Read the model definition and answer for the solid it produces. Units are mm, in the model's axes. A direction names the side the tool comes from. Coordinates: 2 decimals unless noted, no trailing zeros. Order: outer loops, then holes, each group sorted by start corner. A loop starts at its lowest first (then second) coordinate and runs counter-clockwise, first axis right, second up. Notation, with made-up numbers: M -10,24.5 L 20,24.5 A24 cw 20,38.5 Z; hole C -30,31.5 d8. An arc over 180 degrees is marked long. Put each result on its own line as item: value.
from build123d import *

# Parameters (mm, degrees)
F0_R         = 5.25
F1_DEPTH     = 30
F2_DEPTH     = 15
F3_DEPTH     = 30
F4_R         = 2
F6_DEPTH     = 22
F4_R_2       = 3.5
F7_DEPTH     = 4
F5_R         = 2
F8_DEPTH     = 4
F9_W         = 1
F9_H         = 30
F10_DEPTH    = 15
F11_T1_DEPTH = 80
F12_T1_DEPTH = 35.7073493424


# Not quite as in the source:
# - a fillet or chamfer that OpenCascade refuses, or shapes differently, is made with other operations: its cross-section is extruded or revolved along the edge and cut away or added


with BuildPart() as f1:
    # F0 (on Top) → F1 (new body)
    with BuildSketch(Plane.XY):
        with BuildLine():
            ThreePointArc((-11, 0), (0, -11), (11, 0))
            ThreePointArc((11, 0), (7.7781745931, 7.7781745931), (0, 11))
            ThreePointArc((0, 11), (-7.7781745931, 7.7781745931), (-11, 0))
        make_face()
        Circle(F0_R, mode=Mode.SUBTRACT)
        Circle(F0_R)
        with BuildLine():
            ThreePointArc((-1.5811388301, -2.25), (-1.2677476518, 2.4403515918), (2.75, 0))
            ThreePointArc((2.75, 0), (2.4403515918, -1.2677476518), (1.5811388301, -2.25))
            ThreePointArc((1.5811388301, -2.25), (0, -2.75), (-1.5811388301, -2.25))
        make_face(mode=Mode.SUBTRACT)
        with BuildLine():
            ThreePointArc((-11, 0), (-7.7781745931, 7.7781745931), (0, 11))
            Line((0, 11), (-11, 11))
            Line((-11, 11), (-11, 0))
        make_face()
        with BuildLine():
            ThreePointArc((0, 11), (7.7781745931, 7.7781745931), (11, 0))
            Line((11, 0), (11, 11))
            Line((11, 11), (0, 11))
        make_face()
        Polygon((-11, 11), (0, 11), (11, 11), (11, 13), (-11, 13), align=None)
        with BuildLine():
            Line((0, -2.25), (-1.5811388301, -2.25))
            ThreePointArc((-1.5811388301, -2.25), (0, -2.75), (1.5811388301, -2.25))
            Line((1.5811388301, -2.25), (0, -2.25))
        make_face()
        with BuildLine():
            ThreePointArc((1.5811388301, -2.25), (2.4403515918, -1.2677476518), (2.75, 0))
            ThreePointArc((2.75, 0), (-1.2677476518, 2.4403515918), (-1.5811388301, -2.25))
            Line((-1.5811388301, -2.25), (0, -2.25))
            Line((0, -2.25), (1.5811388301, -2.25))
        make_face()
    extrude(amount=F1_DEPTH)

    # F0 (on Top) → F2 (cut)
    with BuildSketch(Plane.XY):
        Circle(F0_R)
        with BuildLine():
            ThreePointArc((-1.5811388301, -2.25), (-1.2677476518, 2.4403515918), (2.75, 0))
            ThreePointArc((2.75, 0), (2.4403515918, -1.2677476518), (1.5811388301, -2.25))
            ThreePointArc((1.5811388301, -2.25), (0, -2.75), (-1.5811388301, -2.25))
        make_face(mode=Mode.SUBTRACT)
        with BuildLine():
            Line((0, -2.25), (-1.5811388301, -2.25))
            ThreePointArc((-1.5811388301, -2.25), (0, -2.75), (1.5811388301, -2.25))
            Line((1.5811388301, -2.25), (0, -2.25))
        make_face()
    extrude(amount=F2_DEPTH, mode=Mode.SUBTRACT)

    # F0 (on Top) → F3 (cut)
    with BuildSketch(Plane.XY):
        with BuildLine():
            ThreePointArc((1.5811388301, -2.25), (2.4403515918, -1.2677476518), (2.75, 0))
            ThreePointArc((2.75, 0), (-1.2677476518, 2.4403515918), (-1.5811388301, -2.25))
            Line((-1.5811388301, -2.25), (0, -2.25))
            Line((0, -2.25), (1.5811388301, -2.25))
        make_face()
    extrude(amount=F3_DEPTH, mode=Mode.SUBTRACT)

    # F4 (on face) → F6 (cut)
    with BuildSketch(Plane(origin=(-11, 0, 0), x_dir=(0, -1, 0), z_dir=(-1, 0, 0))):
        with Locations((-8, 7)):
            Circle(F4_R)
        with Locations((-8, 23)):
            Circle(F4_R)
    extrude(amount=-F6_DEPTH, mode=Mode.SUBTRACT)

    # F4 (on face) → F7 (cut)
    with BuildSketch(Plane(origin=(-11, 0, 0), x_dir=(0, -1, 0), z_dir=(-1, 0, 0))):
        with Locations((-8, 7)):
            Circle(F4_R_2)
        with Locations((-8, 7)):
            Circle(F4_R, mode=Mode.SUBTRACT)
        with Locations((-8, 23)):
            Circle(F4_R_2)
        with Locations((-8, 23)):
            Circle(F4_R, mode=Mode.SUBTRACT)
    extrude(amount=-F7_DEPTH, mode=Mode.SUBTRACT)

    # F5 (on face) → F8 (cut)
    with BuildSketch(Plane.YZ.offset(11)):
        Polygon((6.3545517328, 4.15), (9.6454482672, 4.15), (11.2908965344, 7), (9.6454482672, 9.85), (6.3545517328, 9.85), (4.7091034656, 7), align=None)
        with Locations((8, 7)):
            Circle(F5_R, mode=Mode.SUBTRACT)
        Polygon((6.3545517328, 20.15), (9.6454482672, 20.15), (11.2908965344, 23), (9.6454482672, 25.85), (6.3545517328, 25.85), (4.7091034656, 23), align=None)
        with Locations((8, 23)):
            Circle(F5_R, mode=Mode.SUBTRACT)
    extrude(amount=-F8_DEPTH, mode=Mode.SUBTRACT)

    # F9 (on face) → F10 (cut)
    with BuildSketch(Plane(origin=(0, 13, 0), x_dir=(-1, 0, 0), z_dir=(0, 1, 0))):
        with Locations((0.5, 15)):
            Rectangle(F9_W, F9_H)
        with Locations((-0.5, 15)):
            Rectangle(F9_W, F9_H)
    extrude(amount=-F10_DEPTH, mode=Mode.SUBTRACT)

    # F11: fillet of radius 10 on 2 edges, made by hand

    # F11_s2 → F11_t1 (cut)
    with BuildSketch(Plane.XY.offset(-25)):
        with BuildLine():
            ThreePointArc((-1, 13), (-8.0710678119, 10.0710678119), (-11, 3))
            Line((-11, 3), (-11, 13))
            Line((-11, 13), (-1, 13))
        make_face()
        with BuildLine():
            ThreePointArc((1, 13), (8.0710678119, 10.0710678119), (11, 3))
            Line((11, 3), (11, 13))
            Line((11, 13), (1, 13))
        make_face()
    extrude(amount=F11_T1_DEPTH, mode=Mode.SUBTRACT)

    # F12: chamfer of 1 on 2 edges, made by hand

    # F12_s2 → F12_t1 (cut)
    with BuildSketch(Plane.XY.offset(-2.8536746712)):
        with BuildLine():
            Line((-1, 11.94427191), (-2.1111111111, 12.9380799))
            ThreePointArc((-2.1111111111, 12.9380799), (-1.5705391213, 12.983710989), (-1, 13))
            Line((-1, 13), (-1, 11.94427191))
        make_face()
        with BuildLine():
            Line((2.1111111111, 12.9380799), (1, 11.94427191))
            Line((1, 11.94427191), (1, 13))
            ThreePointArc((1, 13), (1.5705391213, 12.983710989), (2.1111111111, 12.9380799))
        make_face()
    extrude(amount=F12_T1_DEPTH, mode=Mode.SUBTRACT)


solid = f1.part
Q1. Find section B-B on x = 3.5. Write down the section's boundary in (y, z), plus the area to 3 significant figures.
Answers below:
outline: M -10.43,0 L -3.91,0 L -3.91,15 L 3.91,15 L 3.91,0 L 12.68,0 L 12.68,30 L -10.43,30 Z; hole C 8,7 d4; hole C 8,23 d4
area: 551 mm^2
Q2. Given pin 1 (1 mm diameter, centred on x = -3, z = 5.5, fed in from -Y); pin 2 (5 mm diameter, centred on y = 8, z = 23, fed in from +X); pin 3 (2 mm diameter, centred on x = -6, z = 6, fed in from -Y), each flat-ended and moving along its own axis, determine where each tip first touches the part or whether it passes through.
Answers below:
pin 1: stops at y = -10.71
pin 2: stops at x = 7
pin 3: stops at y = -9.8
Q3. Consider line 1 along Z through (x, y) = (-4.55, 8); line 2 along Z through (x, y) = (-8.95, 8); line 3 along X through (y, z) = (10.75, 6.5). Determine where each line is inside the solid, lowest interval first.
Answers below:
line 1: z = 0 to 5, 9 to 21, 25 to 30
line 2: z = 0 to 3.5, 10.5 to 19.5, 26.5 to 30
line 3: x = -7 to -1, 1 to 7
Q4. Find section D-D on y = 2. Write down the section's boundary in (x, z), plus the area to 3 significant figures.
Answers below:
outline: M -11,0 L -4.85,0 L -4.85,15 L -1.89,15 L -1.89,30 L -11,30 Z; M 1.89,15 L 4.85,15 L 4.85,0 L 11,0 L 11,30 L 1.89,30 Z
area: 458 mm^2
Q5. Find section C-C on z = 11. Write down the section's boundary in (x, y), plus the area to 3 significant figures.
Answers below:
outline: M -11,0 A11 ccw 11,0 L 11,3 A10 ccw 2.11,12.94 L 1,11.94 L 1,5.15 A5.25 cw long -1,5.15 L -1,11.94 L -2.11,12.94 A10 ccw -11,3 Z
area: 330 mm^2
Q6. A tool of negligible diameter and unlimited length cuts with its end or side. For faces 1 (the face through (7.583, 10.182, 8.921)), 2 (the face through (-7, 6, 21)), 3 (the face through (-0.217, -5.246, 7.395)), from which of +Z, -Z, +X, -X, +Y, -Y can it reach the whole face along a straight path? Write none if from no direction.
Answers below:
face 1: +X
face 2: -X
face 3: -Z
Q7. For a pull along X with two mould halves and no side action, classify faces 4 (the face through (3.958, 9.474, 8.352)), 5 (the face through (-8.39, 9.74, 14.79)), 6 (the face through (2.3, -2.3, 15)) as +X half, -X half, draft (parallel to the pull), parting line (faces both ways), or undercut.
Answers below:
face 4: draft
face 5: -X half
face 6: undercut
Q8. Find section A-A on z = 6. Write down the section's boundary in (x, y).
Answers below:
outline: M -11,0 A11 ccw 11,0 L 11,3 A10 ccw 10.74,5.29 L 7,5.29 L 7,6.27 L 1,6.27 L 1,5.15 A5.25 cw long -1,5.15 L -1,6.27 L -7,6.27 L -7,4.65 L -10.86,4.65 A10 ccw -11,3 Z; M -7,9.73 L -1,9.73 L -1,11.94 L -2.11,12.94 A10 ccw -7,11 Z; M 1,9.73 L 7,9.73 L 7,10.71 L 7.36,10.71 A10 ccw 2.11,12.94 L 1,11.94 Z
